from build123d import *

# Parameters (mm, degrees)
CROQUIS9_R                      = 6.45
CORTAR_EXTRUIR1_DEPTH           = 2.5
CORTAR_EXTRUIR1_DRAFT           = -45
CORTAR_EXTRUIR1_PROFILE_2_DEPTH = 2.5
CORTAR_EXTRUIR1_PROFILE_2_DRAFT = -45
CORTAR_EXTRUIR1_PROFILE_3_DEPTH = 2.5
CORTAR_EXTRUIR1_PROFILE_3_DRAFT = -45
CORTAR_EXTRUIR1_PROFILE_4_DEPTH = 2.5
CORTAR_EXTRUIR1_PROFILE_4_DRAFT = -45
CORTAR_EXTRUIR1_PROFILE_5_DEPTH = 2.5
CORTAR_EXTRUIR1_PROFILE_5_DRAFT = -45
CORTAR_EXTRUIR1_PROFILE_6_DEPTH = 2.5
CORTAR_EXTRUIR1_PROFILE_6_DRAFT = -45
CROQUIS10_R                     = 39
CROQUIS10_R_2                   = 35
SALIENTE_EXTRUIR1_DEPTH         = 2.5


with BuildPart() as part:
    # Croquis5 → Revolución2 (revolve)
    with BuildSketch(Plane(origin=(0, 0, 0), x_dir=(0, 0, -1), z_dir=(1, 0, 0))):
        Polygon((39, 12.5), (39, -12.5), (88.5, -12.5), (88.5, -8.959553514), (73.5, -3.5), (73.5, 3.5), (88.5, 8.959553514), (88.5, 12.5), align=None)
    revolve(axis=Axis((0, 0, 0), (0, 1, 0)))


with BuildPart() as cortar_extruir1_tool:
    # Croquis9 → Cortar-Extruir1 (with draft: the straight prism first)
    with BuildSketch(Plane(origin=(0, 12.5, 0), x_dir=(1, 0, 0), z_dir=(0, 1, 0))):
        with Locations((58.889727457, 34)):
            Circle(CROQUIS9_R)
    extrude(amount=-CORTAR_EXTRUIR1_DEPTH)
    # Cortar-Extruir1: the draft: its side faces are tilted about the plane it starts from
    cortar_extruir1_sides = [cortar_extruir1_tool.faces().sort_by_distance(p)[0] for p in [
        (52.439727457, 11.25, -34),
    ]]
    draft(cortar_extruir1_sides, Plane(origin=(0, 12.5, 0), x_dir=(1, 0, 0), z_dir=(0, 1, 0)), CORTAR_EXTRUIR1_DRAFT)


with BuildPart() as part_1:
    add(part.part)

    # Cortar-Extruir1: cut by cortar_extruir1_tool
    add(cortar_extruir1_tool.part, mode=Mode.SUBTRACT)


with BuildPart() as cortar_extruir1_profile_2_tool:
    # Croquis9 → Cortar-Extruir1 profile 2 (with draft: the straight prism first)
    with BuildSketch(Plane(origin=(0, 12.5, 0), x_dir=(1, 0, 0), z_dir=(0, 1, 0))):
        with Locations((68, 0)):
            Circle(CROQUIS9_R)
    extrude(amount=-CORTAR_EXTRUIR1_PROFILE_2_DEPTH)
    # Cortar-Extruir1 profile 2: the draft: its side faces are tilted about the plane it starts from
    cortar_extruir1_profile_2_sides = [cortar_extruir1_profile_2_tool.faces().sort_by_distance(p)[0] for p in [
        (61.55, 11.25, 0),
    ]]
    draft(cortar_extruir1_profile_2_sides, Plane(origin=(0, 12.5, 0), x_dir=(1, 0, 0), z_dir=(0, 1, 0)), CORTAR_EXTRUIR1_PROFILE_2_DRAFT)


with BuildPart() as part_2:
    add(part_1.part)

    # Cortar-Extruir1 profile 2: cut by cortar_extruir1_profile_2_tool
    add(cortar_extruir1_profile_2_tool.part, mode=Mode.SUBTRACT)


with BuildPart() as cortar_extruir1_profile_3_tool:
    # Croquis9 → Cortar-Extruir1 profile 3 (with draft: the straight prism first)
    with BuildSketch(Plane(origin=(0, 12.5, 0), x_dir=(1, 0, 0), z_dir=(0, 1, 0))):
        with Locations((58.889727457, -34)):
            Circle(CROQUIS9_R)
    extrude(amount=-CORTAR_EXTRUIR1_PROFILE_3_DEPTH)
    # Cortar-Extruir1 profile 3: the draft: its side faces are tilted about the plane it starts from
    cortar_extruir1_profile_3_sides = [cortar_extruir1_profile_3_tool.faces().sort_by_distance(p)[0] for p in [
        (52.439727457, 11.25, 34),
    ]]
    draft(cortar_extruir1_profile_3_sides, Plane(origin=(0, 12.5, 0), x_dir=(1, 0, 0), z_dir=(0, 1, 0)), CORTAR_EXTRUIR1_PROFILE_3_DRAFT)


with BuildPart() as part_3:
    add(part_2.part)

    # Cortar-Extruir1 profile 3: cut by cortar_extruir1_profile_3_tool
    add(cortar_extruir1_profile_3_tool.part, mode=Mode.SUBTRACT)


with BuildPart() as cortar_extruir1_profile_4_tool:
    # Croquis9 → Cortar-Extruir1 profile 4 (with draft: the straight prism first)
    with BuildSketch(Plane(origin=(0, 12.5, 0), x_dir=(1, 0, 0), z_dir=(0, 1, 0))):
        with Locations((-58.889727457, -34)):
            Circle(CROQUIS9_R)
    extrude(amount=-CORTAR_EXTRUIR1_PROFILE_4_DEPTH)
    # Cortar-Extruir1 profile 4: the draft: its side faces are tilted about the plane it starts from
    cortar_extruir1_profile_4_sides = [cortar_extruir1_profile_4_tool.faces().sort_by_distance(p)[0] for p in [
        (-65.339727457, 11.25, 34),
    ]]
    draft(cortar_extruir1_profile_4_sides, Plane(origin=(0, 12.5, 0), x_dir=(1, 0, 0), z_dir=(0, 1, 0)), CORTAR_EXTRUIR1_PROFILE_4_DRAFT)


with BuildPart() as part_4:
    add(part_3.part)

    # Cortar-Extruir1 profile 4: cut by cortar_extruir1_profile_4_tool
    add(cortar_extruir1_profile_4_tool.part, mode=Mode.SUBTRACT)


with BuildPart() as cortar_extruir1_profile_5_tool:
    # Croquis9 → Cortar-Extruir1 profile 5 (with draft: the straight prism first)
    with BuildSketch(Plane(origin=(0, 12.5, 0), x_dir=(1, 0, 0), z_dir=(0, 1, 0))):
        with Locations((-68, 0)):
            Circle(CROQUIS9_R)
    extrude(amount=-CORTAR_EXTRUIR1_PROFILE_5_DEPTH)
    # Cortar-Extruir1 profile 5: the draft: its side faces are tilted about the plane it starts from
    cortar_extruir1_profile_5_sides = [cortar_extruir1_profile_5_tool.faces().sort_by_distance(p)[0] for p in [
        (-74.45, 11.25, 0),
    ]]
    draft(cortar_extruir1_profile_5_sides, Plane(origin=(0, 12.5, 0), x_dir=(1, 0, 0), z_dir=(0, 1, 0)), CORTAR_EXTRUIR1_PROFILE_5_DRAFT)


with BuildPart() as part_5:
    add(part_4.part)

    # Cortar-Extruir1 profile 5: cut by cortar_extruir1_profile_5_tool
    add(cortar_extruir1_profile_5_tool.part, mode=Mode.SUBTRACT)


with BuildPart() as cortar_extruir1_profile_6_tool:
    # Croquis9 → Cortar-Extruir1 profile 6 (with draft: the straight prism first)
    with BuildSketch(Plane(origin=(0, 12.5, 0), x_dir=(1, 0, 0), z_dir=(0, 1, 0))):
        with Locations((-58.889727457, 34)):
            Circle(CROQUIS9_R)
    extrude(amount=-CORTAR_EXTRUIR1_PROFILE_6_DEPTH)
    # Cortar-Extruir1 profile 6: the draft: its side faces are tilted about the plane it starts from
    cortar_extruir1_profile_6_sides = [cortar_extruir1_profile_6_tool.faces().sort_by_distance(p)[0] for p in [
        (-65.339727457, 11.25, -34),
    ]]
    draft(cortar_extruir1_profile_6_sides, Plane(origin=(0, 12.5, 0), x_dir=(1, 0, 0), z_dir=(0, 1, 0)), CORTAR_EXTRUIR1_PROFILE_6_DRAFT)


with BuildPart() as part_6:
    add(part_5.part)

    # Cortar-Extruir1 profile 6: cut by cortar_extruir1_profile_6_tool
    add(cortar_extruir1_profile_6_tool.part, mode=Mode.SUBTRACT)

    # Croquis10 → Saliente-Extruir1 (add, symmetric)
    with BuildSketch(Plane(origin=(0, 0, 0), x_dir=(1, 0, 0), z_dir=(0, 1, 0))):
        with Locations(Location((0, 0, 0), (0, 0, 90))):
            Circle(CROQUIS10_R)
        with Locations(Location((0, 0, 0), (0, 0, 270))):
            Circle(CROQUIS10_R_2, mode=Mode.SUBTRACT)
    extrude(amount=SALIENTE_EXTRUIR1_DEPTH, both=True)


solid = part_6.part
Source: CAD feature listing. Evaluate the final solid. Frame: model axes, mm. A direction names the side the tool comes from. Give positions to 0.01 mm unless a question says otherwise; leave off trailing zeros. Write each loop counter-clockwise with the first axis right and the second up, starting at its lowest first coordinate (ties: lowest second). Pieces come first, ordered by that corner, then holes. Notation, with made-up numbers: M 66,65 L 91,65 A22 cw 91,85 Z; hole C 5,52 d2. An arc over 180 degrees is marked long. Return JSON: item names as keys, results as strings. Group by question number.
1) Cut plane B-B, the plane x = 0. Output: boundary loops of the cut face in (y, z).
2) Ray query, L1, parallel to Y at x = 35.5, z = -0.5; L2, parallel to Z at x = 11, y = 2.75; L3, parallel to Y at x = 30, z = -77.5. Return the intervals inside material, ascending.
3) Cut plane C-C, the plane y = -0.25. Output: boundary loops of the cut face in (x, z).
4) Set-up query: faces 4 (the face through (-59, 10, 34)), 5 (the face through (18, -12.5, 38)), 6 (the face through (-38.668, -7.57, 5.077)). Return all of +Z, -Z, +X, -X, +Y, -Y with unobstructed straight access to the full face (end or side cutting, diameter ignored); none if empty.
5) First-contact query: pin 1 Ø8.5 at (x, z) = (-67, 1.5) entering from +Y; pin 2 Ø4 at (x, z) = (57, 32) entering from +Y; pin 3 Ø8.5 at (x, z) = (58.5, -33.5) entering from +Y. Flat tips, straight axial feed; report the tip coordinate or a pass-through.
6) Draft query along X for faces 1 (the face through (-1, 12.5, 41)), 2 (the face through (-50.31, 3.84, 54.86)), 3 (the face through (68, 10, 0)). Return one class per face: released by +X, released by -X, zero draft, split by the parting line, or undercut.
Data:
{
 "1": {"outline": "M -12.5,-88.5 L -8.96,-88.5 L -3.5,-73.5 L 3.5,-73.5 L 8.96,-88.5 L 12.5,-88.5 L 12.5,-39 L 2.5,-39 L 2.5,-35 L -2.5,-35 L -2.5,-39 L -12.5,-39 Z; M -12.5,39 L -2.5,39 L -2.5,35 L 2.5,35 L 2.5,39 L 12.5,39 L 12.5,88.5 L 8.96,88.5 L 3.5,73.5 L -3.5,73.5 L -8.96,88.5 L -12.5,88.5 Z"},
 "2": {"L1": "y = -2.5 to 2.5", "L2": "z = -72.67 to -37.42, 37.42 to 72.67", "L3": "y = -12.5 to -7, 7 to 12.5"},
 "3": {"outline": "C 0,0 d147; hole C 0,0 d70"},
 "4": {"face 4": "+Y", "face 5": "+Z, -Z, +X, -X, -Y", "face 6": "-Y"},
 "5": {"pin 1": "stops at y = 12.1", "pin 2": "stops at y = 10.8", "pin 3": "stops at y = 10.93"},
 "6": {"face 1": "zero draft", "face 2": "split by the parting line", "face 3": "undercut"}
}
